Input: part model. Units: mm. Frame: model coordinates. A direction names the side the tool comes from. Give positions to 0.01 mm unless a question says otherwise; leave off trailing zeros. Write each loop counter-clockwise with the first axis right and the second up, starting at its lowest first coordinate (ties: lowest second). Pieces come first, ordered by that corner, then holes.
Autodesk Inventor part; units mm, degrees
ref_plane "BP_POSHUB_ME_XY" through (0, 0, 7) normal (0, 0, 1) x (1, 0, 0)
ref_plane "BP_POSHUB_ME_YZ" through (0, 0, 7) normal (1, 0, 0) x (0, 1, 0)
ref_plane "BP_POSHUB_ME_ZX" through (0, 0, 7) normal (0, 1, 0) x (0, 0, 1)
sketch "Sketch_3" plane through (0, 0, 0) normal (1, 0, 0) x (0, 0, -1)
  line L0 (13, 0) -> (-7, 0)
  line L1 (-7, 0) -> (-7, 19.7)
  line L2 (-7, 19.7) -> (-6.7, 20)
  line L3 (-6.7, 20) -> (-0.3, 20)
  line L4 (-0.3, 20) -> (0, 19.7)
  line L5 (0, 19.7) -> (0, 18.8198)
  line L6 (0, 18.8198) -> (-0.1759, 18.3366)
  arc A0 (-0.1759, 18.3366) -> (0.3035, 17.8134) centre (0.2, 18.1998) ccw
  line L7 (0.3035, 17.8134) -> (1, 18)
  line L8 (1, 18) -> (12, 18)
  line L9 (12, 18) -> (13, 17)
  line L10 (13, 17) -> (13, 0)
  line L11 (13, 0) -> (-7, 0)
revolve "Revolution1" add sketch "Sketch_3" angle 360 about axis through (0, 0, -13) along (0, 0, -1)
sketch "Sketch_1" plane through (0, 0, 0) normal (1, 0, 0) x (0, 0, -1)
  line L0 (13, 0) -> (-7, 0)
  line L1 (-7, 0) -> (-7, 8)
  line L2 (-7, 8) -> (-5.9175, 6.9175)
  line L3 (-5.9175, 6.9175) -> (4.9175, 6.9175)
  line L4 (4.9175, 6.9175) -> (6, 8)
  line L5 (6, 8) -> (6, 8.5)
  line L6 (6, 8.5) -> (12, 8.5)
  line L7 (12, 8.5) -> (13, 9.5)
  line L8 (13, 9.5) -> (13, 0)
  line L9 (13, 0) -> (-7, 0)
revolve "Revolution2" cut sketch "Sketch_1" angle 360 about axis through (0, 0, -13) along (0, 0, -1)
thread "Thread1"
sketch "Sketch_6" plane through (0, 0, 0) normal (1, 0, 0) x (0, 0, -1)
  line L0 (-12, 25) -> (-12, -25)
  line L1 (-12, -25) -> (-2, -25)
  line L2 (-2, -25) -> (-2, -16)
  line L3 (-2, -16) -> (-7, -16)
  line L4 (-7, -16) -> (-7, 16)
  line L5 (-7, 16) -> (-2, 16)
  line L6 (-2, 16) -> (-2, 25)
  line L7 (-2, 25) -> (-12, 25)
extrude "Extrusion1" cut sketch "Sketch_6" along normal mid plane 50
ref_plane "BP_POSHUB_ME_XY" through (0, 0, 7) normal (0, 0, 1) x (1, 0, 0)
ref_plane "BP_POSHUB_ME_YZ" through (0, 0, 7) normal (1, 0, 0) x (0, 1, 0)
ref_plane "BP_POSHUB_ME_ZX" through (0, 0, 7) normal (0, 1, 0) x (0, 0, 1)
ref_plane "DP401_XY" through (0, -16, 7) normal (1, 0, 0) x (0, 0, -1)
ref_plane "DP401_YZ" through (0, -16, 7) normal (0, 0, -1) x (0, 1, 0)
ref_plane "DP401_ZX" through (0, -16, 7) normal (0, 1, 0) x (1, 0, 0)
ref_plane "DPF1_XY" through (0, 20, 2) normal (1, 0, 0) x (0, 0, -1)
ref_plane "DPF1_YZ" through (0, 20, 2) normal (0, 0, -1) x (0, 1, 0)
ref_plane "DPF1_ZX" through (0, 20, 2) normal (0, 1, 0) x (1, 0, 0)
ref_plane "DPF2_XY" through (0, -20, 2) normal (1, 0, 0) x (0, 0, -1)
ref_plane "DPF2_YZ" through (0, -20, 2) normal (0, 0, -1) x (0, 1, 0)
ref_plane "DPF2_ZX" through (0, -20, 2) normal (0, 1, 0) x (1, 0, 0)
ref_plane "DPM2_XY" through (0, 16, 7) normal (1, 0, 0) x (0, 0, -1)
ref_plane "DPM2_YZ" through (0, 16, 7) normal (0, 0, -1) x (0, 1, 0)
ref_plane "DPM2_ZX" through (0, 16, 7) normal (0, 1, 0) x (1, 0, 0)
ref_plane "DPX2_XY" through (0, -16, 7) normal (1, 0, 0) x (0, 0, -1)
ref_plane "DPX2_YZ" through (0, -16, 7) normal (0, 0, -1) x (0, 1, 0)
ref_plane "DPX2_ZX" through (0, -16, 7) normal (0, 1, 0) x (1, 0, 0)
ref_plane "MUTTER_XY" through (0, 0, 7) normal (0, 0, -1) x (1, 0, 0)
ref_plane "MUTTER_YZ" through (0, 0, 7) normal (1, 0, 0) x (0, -1, 0)
ref_plane "MUTTER_ZX" through (0, 0, 7) normal (0, -1, 0) x (0, 0, -1)
ref_plane "SCHRAUBE_XY" through (0, 0, -13) normal (0, 0, 1) x (1, 0, 0)
ref_plane "SCHRAUBE_YZ" through (0, 0, -13) normal (1, 0, 0) x (0, 1, 0)
ref_plane "SCHRAUBE_ZX" through (0, 0, -13) normal (0, 1, 0) x (0, 0, 1)
ref_plane "SCHUBSTANGE_XY" through (0, 0, 0) normal (0, 0, 1) x (1, 0, 0)
ref_plane "SCHUBSTANGE_YZ" through (0, 0, 0) normal (1, 0, 0) x (0, 1, 0)
ref_plane "SCHUBSTANGE_ZX" through (0, 0, 0) normal (0, 1, 0) x (0, 0, 1)
ref_plane "STOPFEN_XY" through (0, 0, 7) normal (0, 0, -1) x (1, 0, 0)
ref_plane "STOPFEN_YZ" through (0, 0, 7) normal (1, 0, 0) x (0, -1, 0)
ref_plane "STOPFEN_ZX" through (0, 0, 7) normal (0, -1, 0) x (0, 0, -1)
properties part number "SLZ_63_Stopfen#"
Q1. Access query for faces 5 (the cylindrical face through (17.847, -2.343, -6.577)), 6 (the flat face through (0, -16, 4)), 7 (the flat face through (0, 18, 2)). Directions: +Z, -Z, +X, -X, +Y, -Y. A direction counts if a zero-diameter tool reaches every point of the face in a straight line with its end or side. Return the directions, or none.
Q2. Mould query, pull axis Y, two halves, no side actions, for faces 1 (the conical face through (-19.82, -0.26, 6.88)), 2 (the cylindrical face through (0.3, -6.91, 0.42)), 3 (the cylindrical face through (7.167, 4.57, -9.042)), 4 (the flat face through (5, 7, 7)). Classes: +Y half, -Y half, draft (parallel to the pull), parting line (faces both ways), or undercut.
Q3. Material intervals for line 1 along X through (y, z) = (0, 2.5); line 2 along X through (y, z) = (0, -9); line 3 along Z through (x, y) = (-4.5, -7), sorted ascending.
Q4. Pin query (flat end, axial travel): pin 1 (1 mm diameter, centred on x = 7, z = -7.5, fed in from -Y); pin 2 (1.5 mm diameter, centred on y = 4.5, z = -5, fed in from -X); pin 3 (10 mm diameter, centred on x = 9.5, z = 2, fed in from +Y). Return the tip coordinate at first contact, or that it passes through.
Q5. Section B-B, the plane z = -9. Return the cut outline in (x, y).
Solutions:
1. face 5: -Z
1. face 6: +Z, +X, -X, -Y
1. face 7: +Z, +X, -X, +Y
2. face 1: parting line
2. face 2: undercut
2. face 3: undercut
2. face 4: draft
3. line 1: x = -20 to -6.92, 6.92 to 20
3. line 2: x = -18 to -8.5, 8.5 to 18
3. line 3: z = -6 to 7
4. pin 1: stops at y = -16.79
4. pin 2: stops at x = -17.61
4. pin 3: stops at y = 19.49
5. outline: circle Ø36 at (0, 0); hole circle Ø17 at (0, 0)
